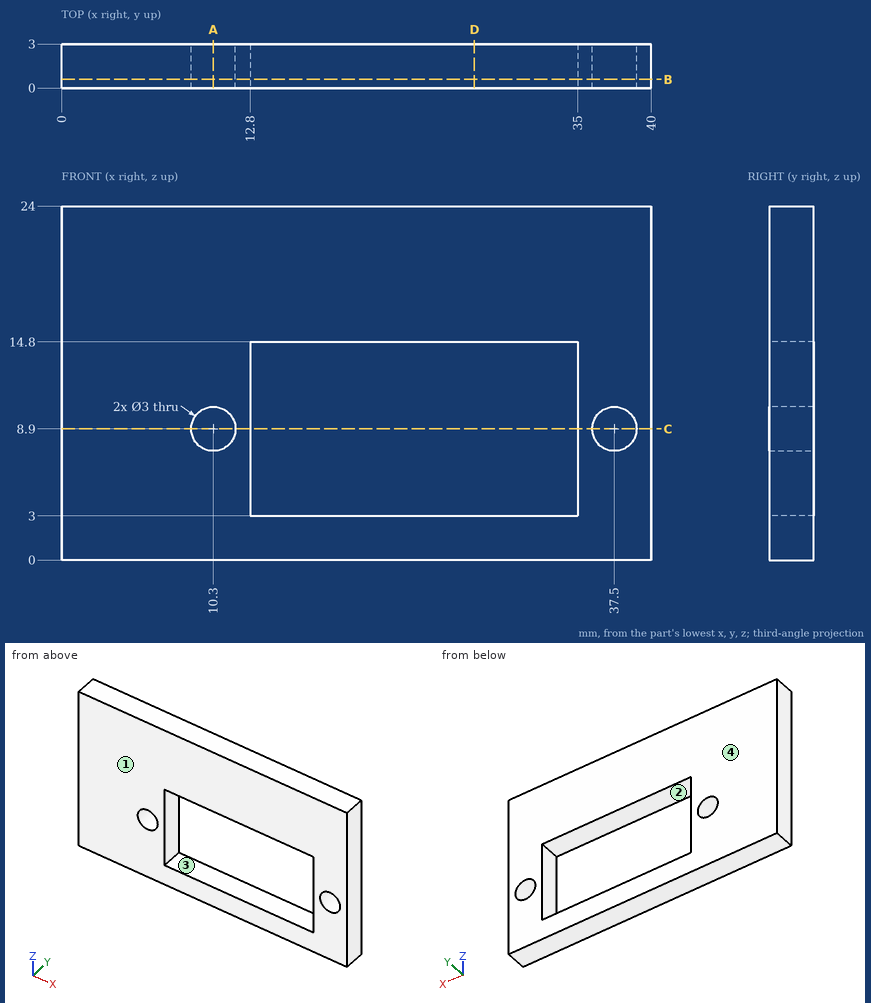
For this review, use the dimensioned drawing (mm, ordinates from the lowest corner) and the shaded views. A direction names the side the tool comes from. Coordinates: 2 decimals unless noted, no trailing zeros. Write each loop counter-clockwise with the first axis right and the second up, starting at its lowest first coordinate (ties: lowest second). Pieces come first, ordered by that corner, then holes. Notation, with made-up numbers: (85, 70.5) - (127, 70.5) arc R34 cw to (127, 103.5) - close; hole circle Ø1 at (-15, 49.25). An arc over 180 degrees is marked (long way). Answer as a JSON object with one key per item and string values. Group by question number.
1. Add section A-A (x = 10.3). Give the boundary of the cut face in (y, z), plus the area to 3 significant figures.
2. Mouldability with a two-part tool opening along X and no side actions: class the marked faces 3 and 4 as pulls with the +X half, pulls with the -X half, needs draft (parallel to the pull), parting line crosses it, or undercut.
3. Add section C-C (z = 8.9). Give the boundary of the cut face in (x, y).
4. Add section D-D (x = 28). Give the boundary of the cut face in (y, z), plus the area to 3 significant figures.
5. Machinability: for the marked faces 1 and 2, which of the approach directions +Z, -Z, +X, -X, +Y, -Y give a long, thin tool a straight path to every point of the face, cutting with its end or side? Answer none if there is none.
6. Add section B-B (y = 0.6). Give the boundary of the cut face in (x, z).
7. To check wall thickness, follow probe 1 along X at (y, z) = (2, 8.9); probe 2 along Z at (x, y) = (31, 1.9); probe 3 along X at (y, z) = (2.1, 14.5). State the ranges of each line that lie inside material, in increasing order.
Findings:
{
 "1": {"outline": "(0, 0) - (3, 0) - (3, 7.4) - (0, 7.4) - close; (0, 10.4) - (3, 10.4) - (3, 24) - (0, 24) - close", "area": "63.0 mm²"},
 "2": {"face 3": "undercut", "face 4": "needs draft"},
 "3": {"outline": "(0, 0) - (8.8, 0) - (8.8, 3) - (0, 3) - close; (11.8, 0) - (12.8, 0) - (12.8, 3) - (11.8, 3) - close; (35, 0) - (36, 0) - (36, 3) - (35, 3) - close; (39, 0) - (40, 0) - (40, 3) - (39, 3) - close"},
 "4": {"outline": "(0, 0) - (3, 0) - (3, 3) - (0, 3) - close; (0, 14.8) - (3, 14.8) - (3, 24) - (0, 24) - close", "area": "36.6 mm²"},
 "5": {"face 1": "+Z, -Z, +X, -X, -Y", "face 2": "+Y, -Y"},
 "6": {"outline": "(0, 0) - (40, 0) - (40, 24) - (0, 24) - close; hole circle Ø3 at (10.3, 8.9); hole (12.8, 3) - (35, 3) - (35, 14.8) - (12.8, 14.8) - close; hole circle Ø3 at (37.5, 8.9)"},
 "7": {"probe 1": "0 to 8.8, 11.8 to 12.8, 35 to 36, 39 to 40", "probe 2": "0 to 3, 14.8 to 24", "probe 3": "0 to 12.8, 35 to 40"}
}
